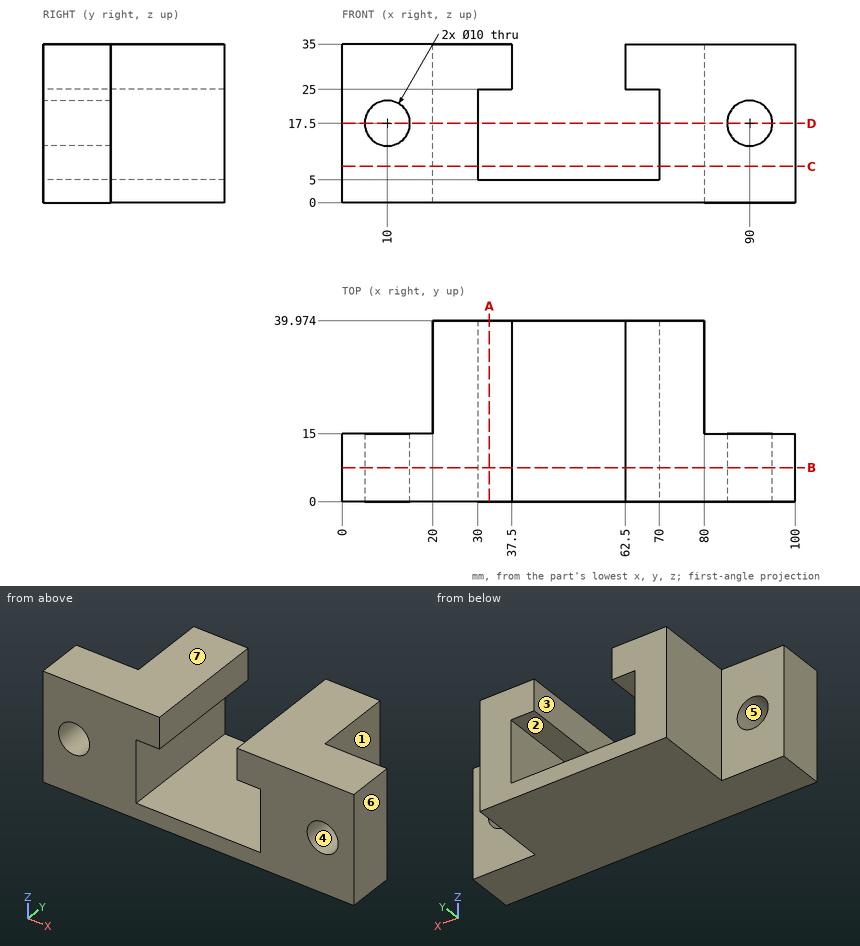
Geometry: see drawing. Coordinates: mm, zero at the bounding-box minimum. A direction names the side the tool comes from. Coordinates: 2 decimals unless noted, no trailing zeros. Loops run counter-clockwise (first coordinate to the right, second up) from the corner with the lowest first, then second, coordinate; pieces in that order, holes last. Notation, with made-up numbers: M 5,-13 L 52,-13 A22 cw 52,-7 Z; hole C 65,8.5 d1. An arc over 180 degrees is marked long. Put each result on its own line as item: value. Start each with the question number.
1) Contact query for flat-ended pins moving along their axis: pin 1 Ø8 at (x, y) = (68, 15) entering from -Z; pin 2 Ø7.5 at (y, z) = (32, 21) entering from +X; pin 3 Ø8 at (y, z) = (26.5, 28.5) entering from -X; pin 4 Ø10 at (x, z) = (87, 18) entering from +Y. Output: stop coordinate, or through.
2) Cut plane C-C on z = 8. Return the cut outline in (x, y).
3) Cut plane B-B on y = 7.5. Return the cut outline in (x, z), then the cut area to 3 significant figures.
4) Ray query, L1, parallel to Z at x = 30.5, y = 5; L2, parallel to Z at x = 10, y = 4.5; L3, parallel to X at y = 30, z = 32. Return the intervals inside material, ascending. Write a range as from..to.
5) Cut plane D-D on z = 17.5. Return the cut outline in (x, y), then the cut area to 3 significant figures.
6) Reachability of the marked faces 1, 2 and 3 from +Z, -Z, +X, -X, +Y, -Y: full face, straight path, thin tool, end or side. Return the list, or none.
7) Cut plane A-A on x = 32.5. Return the cut outline in (y, z).
8) Pull-direction query (X, two-part tool) for the marked faces 4, 5, 6 and 7; classes: pulls with the +X half, pulls with the -X half, needs draft (parallel to the pull), parting line crosses it, or undercut.
The answers:
1. pin 1: stops at z = 0
1. pin 2: stops at x = 80
1. pin 3: stops at x = 20
1. pin 4: stops at y = 15
2. outline: M 0,0 L 30,0 L 30,39.97 L 20,39.97 L 20,15 L 0,15 Z; M 70,0 L 100,0 L 100,15 L 80,15 L 80,39.97 L 70,39.97 Z
3. outline: M 0,0 L 100,0 L 100,35 L 62.5,35 L 62.5,25 L 70,25 L 70,5 L 30,5 L 30,25 L 37.5,25 L 37.5,35 L 0,35 Z; hole C 10,17.5 d10; hole C 90,17.5 d10
3. area: 2,290 mm²
4. L1: z = 0..5, 25..35
4. L2: z = 0..12.5, 22.5..35
4. L3: x = 20..37.5, 62.5..80
5. outline: M 0,0 L 5,0 L 5,15 L 0,15 Z; M 15,0 L 30,0 L 30,39.97 L 20,39.97 L 20,15 L 15,15 Z; M 70,0 L 85,0 L 85,15 L 80,15 L 80,39.97 L 70,39.97 Z; M 95,0 L 100,0 L 100,15 L 95,15 Z
5. area: 1,100 mm²
6. face 1: +Z, -Z, +X, +Y
6. face 2: +Y, -Y
6. face 3: +Z, +Y, -Y
7. outline: M 0,0 L 39.97,0 L 39.97,5 L 0,5 Z; M 0,25 L 39.97,25 L 39.97,35 L 0,35 Z
8. face 4: undercut
8. face 5: undercut
8. face 6: pulls with the +X half
8. face 7: needs draft
